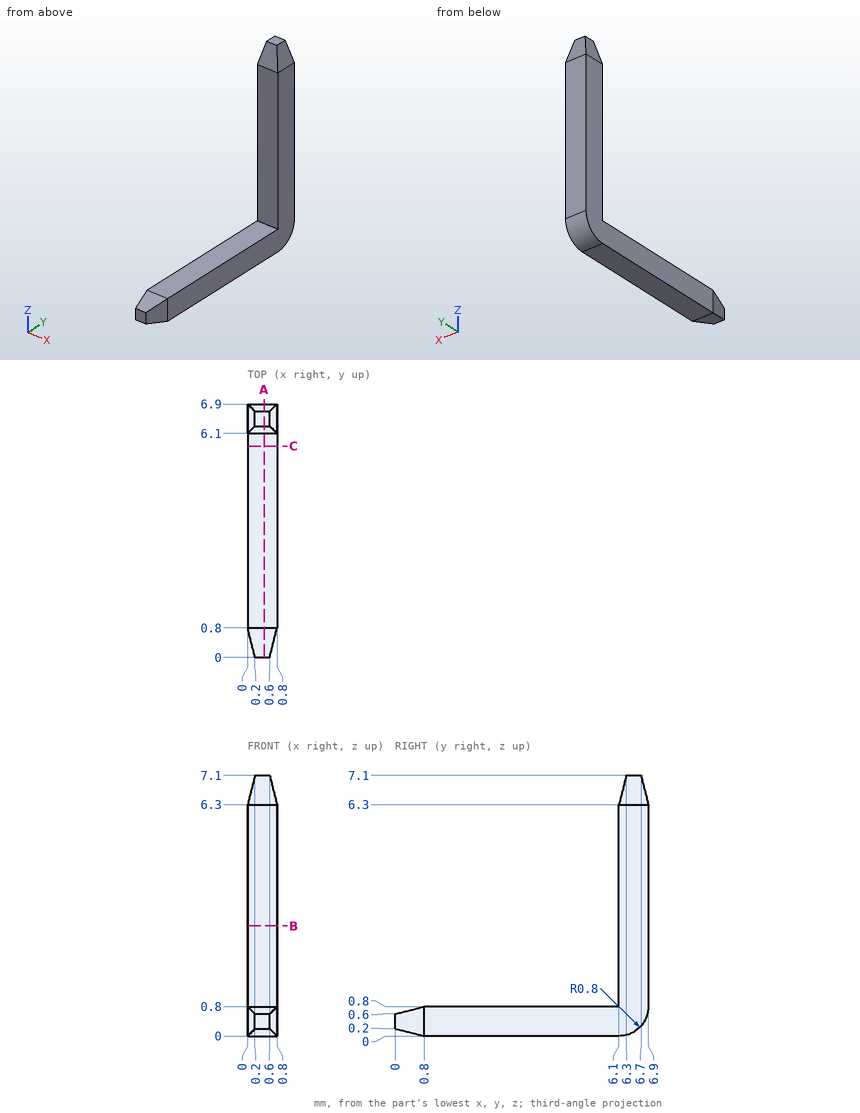
Geometry: see drawing. Coordinates: mm, zero at the bounding-box minimum. Coordinates: 2 decimals unless noted, no trailing zeros. Order: outer loops, then holes, each group sorted by start corner. A loop starts at its lowest first (then second) coordinate and runs counter-clockwise, first axis right, second up. Notation, with made-up numbers: (12, -0.75) -> (69, -0.75) arc R26 cw to (69, 16.25) -> close; hole circle Ø4 at (67, 38.25). An arc over 180 degrees is marked (long way). Write each question's results on one line, items separated by ' | '. Start each with the question number.
1) Material intervals for line 1 along Z through (x, y) = (0.4, 2); line 2 along Y through (x, z) = (0.45, 4.5); line 3 along Z through (x, y) = (0.5, 6.5), sorted ascending.
2) First-contact query: pin 1 (2 mm diameter, centred on y = 4, z = 3, fed in from +X); pin 2 (4 mm diameter, centred on y = 3, z = 1.5, fed in from +X). Flat tips, straight axial feed; report the tip coordinate or a pass-through.
3) Cut plane C-C, the plane y = 5.75. Output: boundary loops of the cut face in (x, z), and give its area (3 significant figures).
4) Cut plane B-B, the plane z = 3. Output: boundary loops of the cut face in (x, y).
5) Cut plane A-A, the plane x = 0.45. Output: boundary loops of the cut face in (y, z), and give its area (3 significant figures).
Checks:
1) line 1: 0 to 0.8 | line 2: 6.1 to 6.9 | line 3: 0.11 to 7.1
2) pin 1: through | pin 2: x = 0.8
3) outline: (0, 0) -> (0.8, 0) -> (0.8, 0.8) -> (0, 0.8) -> close | area: 0.640 mm^2
4) outline: (0, 6.1) -> (0.8, 6.1) -> (0.8, 6.9) -> (0, 6.9) -> close
5) outline: (0, 0.2) -> (0.8, 0) -> (6.1, 0) arc R0.8 ccw to (6.9, 0.8) -> (6.9, 6.3) -> (6.7, 7.1) -> (6.3, 7.1) -> (6.1, 6.3) -> (6.1, 0.8) -> (0.8, 0.8) -> (0, 0.6) -> close | area: 10.1 mm^2
